Source: CAD feature listing. Evaluate the final solid. Frame: model axes, mm. A direction names the side the tool comes from. Round coordinates to 2 decimals unless told otherwise and drop trailing zeros. Order: outer loops, then holes, each group sorted by start corner. A loop starts at its lowest first (then second) coordinate and runs counter-clockwise, first axis right, second up. Notation, with made-up numbers: (57, 37) - (72, 37) arc R5 cw to (72, 46) - close; hole circle Ø9 at (69, 57.25). An arc over 180 degrees is marked (long way). Return JSON: item names as keys, results as strings. Group by question number.
1) Section A-A, the plane z = 26. Return loops of the section in (x, y), plus the area to 3 significant figures.
2) Section C-C, the plane z = 2.75. Return loops of the section in (x, y), plus the area to 3 significant figures.
3) Contact query for flat-ended pins moving along their axis: P1, Ø2, axis at y = 3.5, z = 13, coming from the -X side; P2, Ø2, axis at y = 1, z = 7.5, coming from the +X side; P3, Ø2.5, axis at x = 0, y = 2.3, coming from the -Z side. Output: stop coordinate, or through.
4) Mould query, pull axis X, two halves, no side actions, for faces 1 (the flat face through (0, 2, 2)), 2 (the flat face through (0, 4.6, 14)), 3 (the flat face through (-2.01, 3.43, 13.85)), 4 (the cylindrical face through (1.5, 2.37, 0.99)). Classes: pulls with the +X half, pulls with the -X half, needs draft (parallel to the pull), parting line crosses it, or undercut.
5) Ray query, line 1 (Y direction, x = 0, z = 1.15); line 2 (Z direction, x = -1.45, y = 2.15); line 3 (X direction, y = 1.25, z = 6.5). Return the intervals inside material, ascending. Write a range as from..to.
6) Section B-B, the plane x = 0. Return loops of the section in (y, z), plus the area to 3 significant figures.
7) Access query for faces 5 (the flat face through (0, 2, 25.1)), 6 (the flat face through (0, 4, 0)). Directions: +Z, -Z, +X, -X, +Y, -Y. A direction counts if a zero-diameter tool reaches every point of the face in a straight line with its end or side. Return the directions, or none.
8) Section D-D, the plane y = 4.35. Return loops of the section in (x, z), plus the area to 3 significant figures.
```python
from build123d import *

# Parameters (mm, degrees)
BOSS_EXTRUDE1_DEPTH = 28.1
SKETCH2_R           = 1.5
CUT_EXTRUDE1_DEPTH  = 2
CUT_EXTRUDE2_START  = -3
SKETCH3_R           = 1.5
CUT_EXTRUDE2_DEPTH  = 3


with BuildPart() as part:
    # Sketch1 → Boss-Extrude1 (new body)
    with BuildSketch(Plane.XY):
        Polygon((-1.4, 4.6), (1.4, 4.6), (2.599787383, 2.3), (1.4, 0), (-1.4, 0), (-2.599787383, 2.3), align=None)
    extrude(amount=BOSS_EXTRUDE1_DEPTH)

    # Sketch2 → Cut-Extrude1 (cut)
    with BuildSketch(Plane(origin=(0, 0, 0), x_dir=(-1, 0, 0), z_dir=(0, 0, -1))):
        with Locations((0, 2.3)):
            Circle(SKETCH2_R)
    extrude(amount=-CUT_EXTRUDE1_DEPTH, mode=Mode.SUBTRACT)

    # Sketch3 → Cut-Extrude2 (cut)
    with BuildSketch(Plane.XY.offset(28.1).offset(CUT_EXTRUDE2_START)):
        with Locations(Location((0, 2.3, 0), (0, 0, 180))):
            Circle(SKETCH3_R)
    extrude(amount=CUT_EXTRUDE2_DEPTH, mode=Mode.SUBTRACT)


solid = part.part
```
Geometry check:
{
 "1": {"outline": "(-2.6, 2.3) - (-1.4, 0) - (1.4, 0) - (2.6, 2.3) - (1.4, 4.6) - (-1.4, 4.6) - close; hole circle Ø3 at (0, 2.3)", "area": "11.3 mm2"},
 "2": {"outline": "(-2.6, 2.3) - (-1.4, 0) - (1.4, 0) - (2.6, 2.3) - (1.4, 4.6) - (-1.4, 4.6) - close", "area": "18.4 mm2"},
 "3": {"P1": "x = -2.5", "P2": "x = 2.44", "P3": "z = 2"},
 "4": {"face 1": "undercut", "face 2": "needs draft", "face 3": "pulls with the -X half", "face 4": "undercut"},
 "5": {"line 1": "0..0.8, 3.8..4.6", "line 2": "2..25.1", "line 3": "-2.05..2.05"},
 "6": {"outline": "(0, 0) - (0.8, 0) - (0.8, 2) - (3.8, 2) - (3.8, 0) - (4.6, 0) - (4.6, 28.1) - (3.8, 28.1) - (3.8, 25.1) - (0.8, 25.1) - (0.8, 28.1) - (0, 28.1) - close", "area": "114 mm2"},
 "7": {"face 5": "+Z", "face 6": "-Z, +X, -X, +Y, -Y"},
 "8": {"outline": "(-1.53, 0) - (1.53, 0) - (1.53, 28.1) - (-1.53, 28.1) - close", "area": "86.0 mm2"}
}
